Autodesk Inventor part; units mm, degrees
ref_plane "YZ Plane" through (0, 0, 0) normal (1, 0, 0) x (0, 1, 0)
ref_plane "XZ Plane" through (0, 0, 0) normal (0, 1, 0) x (-1, 0, 0)
ref_plane "XY Plane" through (0, 0, 0) normal (0, 0, 1) x (1, 0, 0)
sketch "Sketch1" plane through (0, 0, 0) normal (1, 0, 0) x (0, 1, 0)
  arc A0 (0, -15.5) -> (0, 15.5) centre (0, 0) ccw
  line L0 (0, -15.5) -> (-10, -15.5)
  line L1 (0, -15.5) -> (0, -16.75)
  arc A1 (0, -16.75) -> (0, 16.75) centre (0, 0) ccw
  line L2 (0, -16.75) -> (-10, -16.75)
  line L3 (-10, -15.5) -> (-10, -27.5)
  line L4 (-10, -16.75) -> (-8.75, -16.75)
  line L5 (-8.75, -27.5) -> (-8.75, -28.75)
  line L6 (-15.5, 0) -> (-15.5, -28.75)
  line L7 (-8.75, -27.5) -> (-8.75, -16.75)
  line L8 (0, 0) -> (-6.7436, 0)
  line L9 (0, 15.5) -> (-10, 15.5)
  line L10 (0, 16.75) -> (-8.75, 16.75)
  line L11 (-10, 15.5) -> (-10, 27.5)
  line L12 (-8.75, 27.5) -> (-8.75, 28.75)
  line L13 (-15.5, 0) -> (-15.5, 28.75)
  line L14 (-8.75, 27.5) -> (-8.75, 16.75)
  line L15 (-10, -27.5) -> (-10, -28.5)
  line L16 (-10, -28.5) -> (-15.5, -28.5)
  line L17 (-15.5, -28.5) -> (-15.5, -29.75)
  line L18 (-15.5, -29.75) -> (-8.75, -29.75)
  line L19 (-8.75, -29.75) -> (-8.75, -28.75)
  line L20 (-8.75, 27.5) -> (-8.75, 28.75)
  line L21 (-10, 27.5) -> (-10, 28.5)
  line L22 (-10, 28.5) -> (-15.5, 28.5)
  line L23 (-15.5, 28.5) -> (-15.5, 29.75)
  line L24 (-15.5, 29.75) -> (-8.75, 29.75)
  line L25 (-8.75, 29.75) -> (-8.75, 28.75)
  point P0 (-10, 16.75)
  dimension "d0" = 31
  dimension "d1" = 10
  dimension "d2" = 1.25
  dimension "d3" = 12
  dimension "d4" = 1.25
  dimension "d5" = 1.25
  dimension "d6" = 1
  dimension "d7" = 1.25
extrude "Extrusion1" add sketch "Sketch1" along normal blind 35 contours L1 L2 L3 L0 | A0 L9 L11 L21 L22 L13 L23 L24 L25 L12 L14 L10 A1 L1 | L2 L7 L5 L19 L18 L17 L6 L16 L15 L3
sketch "Sketch2" plane through (35, 0, 0) normal (1, 0, 0) x (0, 0, -1)
  line L0 (29.75, -8.75) -> (16.75, -8.75)
  line L1 (16.75, -8.75) -> (16.75, 0)
  arc A0 (16.75, 0) -> (-16.75, 0) centre (0, 0) ccw
  line L2 (-16.75, 0) -> (-16.75, -8.75)
  line L3 (-16.75, -8.75) -> (-29.75, -8.75)
  line L4 (-29.75, -8.75) -> (-29.75, -15.5)
  line L5 (-29.75, -15.5) -> (-28.5, -15.5)
  line L6 (-28.5, -15.5) -> (-28.5, -10)
  line L7 (-28.5, -10) -> (-15.5, -10)
  line L8 (-15.5, -10) -> (-15.5, 0)
  arc A1 (15.5, 0) -> (-15.5, 0) centre (0, 0) ccw
  line L9 (15.5, 0) -> (15.5, -10)
  line L10 (15.5, -10) -> (28.5, -10)
  line L11 (28.5, -10) -> (28.5, -15.5)
  line L12 (28.5, -15.5) -> (29.75, -15.5)
  line L13 (29.75, -15.5) -> (29.75, -8.75)
  line L14 (-28.5, -15.5) -> (-28.5, -10)
  line L15 (-28.5, -15.5) -> (0, -15.5)
  line L16 (0, -15.5) -> (0, 27.5)
  line L17 (0, 27.5) -> (0, 6)
  line L18 (21.5, 6) -> (21.5, -15.5)
  line L19 (21.5, -15.5) -> (22.75, -15.5)
  line L20 (22.75, -15.5) -> (22.75, 6)
  line L21 (-21.5, 6) -> (-21.5, -15.5)
  line L22 (-21.5, -15.5) -> (-22.75, -15.5)
  line L23 (-22.75, -15.5) -> (-22.75, 6)
  arc A2 (22.75, 6) -> (-22.75, 6) centre (0, 6) ccw
  arc A3 (-17.3205, -8.75) -> (-16.1729, -10) centre (0, 6) ccw
  arc A4 (16.1729, -10) -> (17.3205, -8.75) centre (0, 6) ccw
  arc A5 (-16.75, -7.4792) -> (-15.5, -8.8997) centre (0, 6) ccw
  arc A6 (15.5, -8.8997) -> (16.75, -7.4792) centre (0, 6) ccw
  arc A7 (21.5, 6) -> (-21.5, 6) centre (0, 6) ccw
  dimension "d10" = 43
  dimension "d11" = 21.5
  dimension "d12" = 1.25
extrude "Extrusion2" add sketch "Sketch2" along normal blind 103 contours L18 A7 L21 L3 L23 A2 L20 L0 | L0 L20 L10 L18 | L10 L20 L19 L18 | L3 L21 L7 L23 | L7 L21 L15 L23
sketch "Sketch3" plane through (35, 0, 0) normal (-1, 0, 0) x (0, 0, 1)
  line L0 (-22.75, -8.75) -> (-21.5, -8.75)
  line L1 (-21.5, 6) -> (-21.5, -8.75)
  arc A0 (21.5, 6) -> (-21.5, 6) centre (0, 6) ccw
  line L2 (21.5, -8.75) -> (21.5, 6)
  line L3 (21.5, -8.75) -> (22.75, -8.75)
  line L4 (22.75, 6) -> (22.75, -8.75)
  arc A1 (22.75, 6) -> (-22.75, 6) centre (0, 6) ccw
  line L5 (-22.75, -8.75) -> (-22.75, 6)
  line L6 (-29.75, -8.75) -> (-16.75, -8.75)
  line L7 (-29.75, -15.5) -> (-29.75, -8.75)
  line L8 (-28.5, -15.5) -> (-29.75, -15.5)
  line L9 (-28.5, -10) -> (-28.5, -15.5)
  line L10 (-15.5, -10) -> (-28.5, -10)
  line L11 (-15.5, 0) -> (-15.5, -10)
  arc A2 (15.5, 0) -> (-15.5, 0) centre (0, 0) ccw
  line L12 (15.5, -10) -> (15.5, 0)
  line L13 (28.5, -10) -> (15.5, -10)
  line L14 (28.5, -15.5) -> (28.5, -10)
  line L15 (29.75, -15.5) -> (28.5, -15.5)
  line L16 (29.75, -8.75) -> (29.75, -15.5)
  line L17 (16.75, -8.75) -> (29.75, -8.75)
  line L18 (16.75, 0) -> (16.75, -8.75)
  arc A3 (16.75, 0) -> (-16.75, 0) centre (0, 0) ccw
  line L19 (-16.75, -8.75) -> (-16.75, 0)
extrude "Extrusion3" add sketch "Sketch3" along normal blind 1.25 contours L5 A1 L4 L3 L2 A0 L1 L0 | L1 A0 L2 L17 L18 A3 L19 L6
sketch "Sketch4" plane through (0, -8.75, 29.75) normal (0, 1, 0) x (1, 0, 0)
  line L0 (33.75, 7) -> (33.75, 13)
  line L1 (0, 13) -> (33.75, 13)
  line L2 (0, 13) -> (0, 0)
  line L3 (0, 0) -> (35, 0)
  line L4 (35, 7) -> (35, 0)
  line L5 (35, 7) -> (33.75, 7)
  line L6 (33.75, 46.5) -> (33.75, 52.5)
  line L7 (33.75, 52.5) -> (35, 52.5)
  line L8 (35, 59.5) -> (35, 52.5)
  line L9 (0, 59.5) -> (35, 59.5)
  line L10 (0, 59.5) -> (0, 46.5)
  line L11 (0, 46.5) -> (33.75, 46.5)
  line L12 (33.75, 7) -> (33.75, 0)
  line L13 (0, 0) -> (35, 0)
  line L14 (33.75, 52.5) -> (33.75, 59.5)
  line L15 (0, 59.5) -> (35, 59.5)
  point P0 (0, 29.75)
extrude "Extrusion4" cut sketch "Sketch4" against normal through all contours L5 L4 L3 L12 | L14 L9 L8 L7
sketch "Sketch5" plane through (35, 0, 0) normal (-1, 0, 0) x (0, 0, 1)
  line L0 (-21.5, -10) -> (-22.75, -10)
  line L1 (-22.75, -15.5) -> (-22.75, -10)
  line L2 (-21.5, -15.5) -> (-22.75, -15.5)
  line L3 (-21.5, -10) -> (-21.5, -15.5)
  line L4 (22.75, -10) -> (21.5, -10)
  line L5 (21.5, -15.5) -> (21.5, -10)
  line L6 (22.75, -15.5) -> (21.5, -15.5)
  line L7 (22.75, -10) -> (22.75, -15.5)
  point P0 (0, 0)
extrude "Extrusion5" add sketch "Sketch5" along normal blind 2.5
sketch "Sketch6" plane through (138, -15.5, 22.75) normal (0, 0, 1) x (1, 0, 0)
  line L0 (-104.25, 0) -> (-104.25, 6.75)
  line L1 (-138, 6.75) -> (-104.25, 6.75)
  line L2 (-138, 6.75) -> (-138, 0)
  line L3 (-138, 0) -> (-104.25, 0)
  line L4 (-105.5, 0) -> (-105.5, 5.5)
  line L5 (-105.5, 5.5) -> (-104.25, 5.5)
  point P0 (-138, 15.5)
extrude "Extrusion6" add sketch "Sketch6" along normal blind 7 contours L3 L4 L5 L0
sketch "Sketch7" plane through (138, -15.5, -22.75) normal (0, 0, -1) x (-1, 0, 0)
  line L0 (104.25, 6.75) -> (104.25, 0)
  line L1 (105.5, 5.5) -> (105.5, 0)
  line L2 (103, 5.5) -> (105.5, 5.5)
  line L3 (105.5, 0) -> (0, 0)
  point P0 (138, 15.5)
  point P1 (104.25, 5.5)
extrude "Extrusion7" add sketch "Sketch7" along normal blind 7
sketch "Sketch8" plane through (138, 0, 0) normal (1, 0, 0) x (0, 0, -1)
  line L0 (-22.75, 6) -> (-22.75, -15.5)
  line L1 (-22.75, -15.5) -> (-21.5, -15.5)
  line L2 (-21.5, -15.5) -> (-21.5, 6)
  arc A0 (21.5, 6) -> (-21.5, 6) centre (0, 6) ccw
  line L3 (21.5, 6) -> (21.5, -15.5)
  line L4 (21.5, -15.5) -> (22.75, -15.5)
  line L5 (22.75, -15.5) -> (22.75, 6)
  arc A1 (22.75, 6) -> (-22.75, 6) centre (0, 6) ccw
  line L6 (-22.75, -15.5) -> (22.75, -15.5)
  line L7 (-21.5, -15.5) -> (-28.5, -15.5)
  point P0 (0, 0)
extrude "Extrusion8" add sketch "Sketch8" along normal blind 1.25
sketch "Sketch9" plane through (33.75, -8.75, 22.75) normal (0, 0, 1) x (1, 0, 0)
  line L0 (0, 0) -> (0, -6.75)
  line L1 (0, -6.75) -> (105.5, -6.75)
  line L2 (105.5, 14.75) -> (105.5, -6.75)
  line L3 (105.5, 14.75) -> (0, 14.75)
  line L4 (0, 0) -> (0, 14.75)
  line L5 (105.5, -6.75) -> (96.5, -6.75)
  line L6 (-1.25, -6.75) -> (104.25, -6.75)
  line L7 (96.5, -6.75) -> (96.5, -5.5)
  line L8 (96.5, -5.5) -> (88.5, -5.5)
  line L9 (88.5, -5.5) -> (88.5, -6.75)
  point P0 (-33.75, 8.75)
  dimension "d27" = 9
  dimension "d28" = 1.25
  dimension "d29" = 8
extrude "Extrusion9" add sketch "Sketch9" along normal blind 8 contours L9 L8 L7 L1
sketch "Sketch10" plane through (33.75, -8.75, -22.75) normal (0, 0, -1) x (-1, 0, 0)
  line L0 (-88.5, -6.75) -> (-96.5, -6.75)
  line L1 (-88.5, -5.5) -> (-88.5, -6.75)
  line L2 (-88.5, -6.75) -> (-96.5, -6.75)
  line L3 (-96.5, -6.75) -> (-96.5, -5.5)
  line L4 (-96.5, -5.5) -> (-88.5, -5.5)
  point P0 (33.75, 8.75)
extrude "Extrusion10" add sketch "Sketch10" along normal blind 8
sketch "Sketch11" plane through (122.25, -14.25, -22.75) normal (0, 1, 0) x (1, 0, 0)
  line L0 (8, 0) -> (0, 0)
  line L1 (8, 0) -> (8, 8)
  line L2 (0, 8) -> (8, 8)
  line L3 (0, 0) -> (0, 8)
  line L4 (0, -45.5) -> (8, -45.5)
  line L5 (0, -45.5) -> (0, -53.5)
  line L6 (8, -53.5) -> (0, -53.5)
  line L7 (8, -45.5) -> (8, -53.5)
  line L8 (0, -45.5) -> (0, -53.5)
  line L9 (0, -53.5) -> (4, -53.5)
  line L10 (0, -53.5) -> (8, -53.5)
  line L11 (4, -53.5) -> (4, -49.5)
  circle A0 centre (4, -49.5) radius 1.8
  line L12 (0, 8) -> (8, 8)
  line L13 (8, 8) -> (4, 8)
  line L14 (8, 8) -> (12, 8) construction
  line L15 (4, 8) -> (4, 4)
  line L16 (0, 0) -> (0, 8)
  circle A1 centre (4, 4) radius 1.8
  point P0 (-122.25, -22.75)
  dimension "d34" = 4
  dimension "d35" = 3.6
  dimension "d36" = 4
  dimension "d37" = 180
  dimension "d38" = 3.6
extrude "Extrusion11" cut sketch "Sketch11" against normal blind 8 contours A1 | A0
fillet "Fillet1" radius 1 6 edges at (130.25, -14.875, 22.75) (126.25, -14.25, 22.75) (122.25, -14.875, 22.75) (130.25, -14.875, -22.75) (126.25, -14.25, -22.75) (122.25, -14.875, -22.75)
fillet "Fillet2" radius 2 3 edges at (33.75, -4.375, -16.75) (33.75, -4.375, 16.75) (33.75, 16.75, 0)
sketch "Sketch12" plane through (0, -8.75, -16.75) normal (0, 1, 0) x (1, 0, 0)
  arc A0 (31.75, 0) -> (33.75, 2) centre (31.75, 2) ccw
  line L0 (33.75, 2) -> (33.75, 6)
  line L1 (33.75, 6) -> (33.75, 13)
  line L2 (0, 13) -> (33.75, 13)
  line L3 (0, 13) -> (0, 0)
  line L4 (0, 0) -> (31.75, 0)
  arc A1 (33.75, -35.5) -> (31.75, -33.5) centre (31.75, -35.5) ccw
  line L5 (0, -33.5) -> (31.75, -33.5)
  line L6 (0, -33.5) -> (0, -46.5)
  line L7 (0, -46.5) -> (33.75, -46.5)
  line L8 (33.75, -46.5) -> (33.75, -39.5)
  line L9 (33.75, -39.5) -> (33.75, -35.5)
  line L10 (0, 13) -> (-2.5, 13)
  line L11 (-2.5, 13) -> (4, 13)
  line L12 (0, 13) -> (33.75, 13)
  line L13 (4, 13) -> (4, 8.75)
  line L14 (4, 8.75) -> (4, 4.4)
  circle A2 centre (4, 4.4) radius 2.55
  line L15 (0, 0) -> (0, -16.75)
  line L16 (0, -16.75) -> (16.875, -16.75)
  circle A3 centre (4, -37.9) radius 2.55
  dimension "d43" = 2.5
  dimension "d44" = 6.5
  dimension "d45" = 4.25
  dimension "d46" = 4.35
  dimension "d47" = 5.1
extrude "Extrusion12" cut sketch "Sketch12" against normal blind 8 contours A2 | A3
properties part number "carcasa_motores"
Verification items for the finished model (mm, model axes). A direction names the side the tool comes from. Coordinates: 2 decimals unless noted, no trailing zeros. Loops run counter-clockwise (first coordinate to the right, second up) from the corner with the lowest first, then second, coordinate; pieces in that order, holes last. Notation, with made-up numbers: (34, -5.75) -> (72, -5.75) arc R19 ccw to (72, 4.25) -> close; hole circle Ø7 at (64, 45). An arc over 180 degrees is marked (long way). Answer as a JSON object with one key per item and string values. Group by question number.
Item 1: Sectioned sample at B-B on x = 4. Record the boundary of the cut face in (y, z), plus the area to 3 significant figures.
Item 2: Sectioned sample at A-A on z = -26.75. Record the boundary of the cut face in (x, y), plus the area to 3 significant figures.
Item 3: Sectioned sample at C-C on y = -3. Record the boundary of the cut face in (x, z), plus the area to 3 significant figures.
Item 4: Scan lines: probe 1 along X at (y, z) = (-9.15, -21.15); probe 2 along Z at (x, y) = (4, -9.7); probe 3 along Z at (x, y) = (126, -15). Record each from-to range of solid material in increasing order.
Item 5: Sectioned sample at D-D on z = 0. Record the boundary of the cut face in (x, y), plus the area to 3 significant figures.
Item 6: Mould release check, pull along X, two halves, no side actions. Record for faces 4 (the flat face through (33.75, -12, -26)), 5 (the cylindrical face through (87.238, 28.744, -0.5)), 6 (the flat face through (139.25, 7, 0)): +X half, -X half, draft (parallel to the pull), parting line (faces both ways), or undercut.
Item 7: Tool access check on faces 1 (the flat face through (17, -12, 29.75)), 2 (the flat face through (17, -5, 15.5)), 3 (the flat face through (16, -4, 16.75)). Record the directions out of +Z, -Z, +X, -X, +Y, -Y that give a thin tool (end or side, any length) a straight path to the whole face; none if there is none.
Item 8: Depth check by flat-ended pin: pin 1 (1 mm diameter, centred on y = 18, z = -9, fed in from -X); pin 2 (1.4 mm diameter, centred on y = -15, z = 28, fed in from +X); pin 3 (4 mm diameter, centred on x = 124, z = 11, fed in from +Y). Enter the tip coordinate at first touch or a pass-through.
Evaluation:
{
 "1": {"outline": "(-15.5, -29.75) -> (-8.75, -29.75) -> (-8.75, -23.7) -> (-10, -23.7) -> (-10, -28.5) -> (-15.5, -28.5) -> close; (-15.5, 28.5) -> (-10, 28.5) -> (-10, 23.7) -> (-8.75, 23.7) -> (-8.75, 29.75) -> (-15.5, 29.75) -> close; (-10, -18.6) -> (-8.75, -18.6) -> (-8.75, -16.75) -> (0, -16.75) arc R16.75 ccw to (0, 16.75) -> (-8.75, 16.75) -> (-8.75, 18.6) -> (-10, 18.6) -> (-10, 15.5) -> (0, 15.5) arc R15.5 cw to (0, -15.5) -> (-10, -15.5) -> close", "area": "122 mm²"},
 "2": {"outline": "(0, -10) -> (32.5, -10) -> (32.5, -15.5) -> (33.75, -15.5) -> (33.75, -8.75) -> (0, -8.75) -> close; (122.25, -15.5) -> (124.45, -15.5) -> (124.45, -14.25) -> (122.25, -14.25) -> close; (128.05, -15.5) -> (130.25, -15.5) -> (130.25, -14.25) -> (128.05, -14.25) -> close", "area": "54.6 mm²"},
 "3": {"outline": "(0, -16.75) -> (31.75, -16.75) arc R2 cw to (33.75, -18.75) -> (33.75, -22.75) -> (139.25, -22.75) -> (139.25, 22.75) -> (33.75, 22.75) -> (33.75, 18.75) arc R2 cw to (31.75, 16.75) -> (0, 16.75) -> (0, 15.5) -> (35, 15.5) -> (35, 21.5) -> (138, 21.5) -> (138, -21.5) -> (35, -21.5) -> (35, -15.5) -> (0, -15.5) -> close", "area": "419 mm²"},
 "4": {"probe 1": "x = 0 to 1.45, 6.55 to 35, 138 to 139.25", "probe 2": "z = -29.75 to -23.7, -18.6 to -15.5, 15.5 to 18.6, 23.7 to 29.75", "probe 3": "z = -30.75 to -28.53, -24.97 to -21.5, 21.5 to 24.97, 28.53 to 30.75"},
 "5": {"outline": "(0, 15.5) -> (35, 15.5) -> (35, 27.5) -> (138, 27.5) -> (138, -15.5) -> (139.25, -15.5) -> (139.25, 28.75) -> (33.75, 28.75) -> (33.75, 18.75) arc R2 cw to (31.75, 16.75) -> (0, 16.75) -> close", "area": "244 mm²"},
 "6": {"face 4": "undercut", "face 5": "draft", "face 6": "+X half"},
 "7": {"face 1": "+Z, -X, +Y, -Y", "face 2": "-X, -Y", "face 3": "+Z, -X, +Y"},
 "8": {"pin 1": "stops at x = 33.75", "pin 2": "stops at x = 130.25", "pin 3": "stops at y = 26.89"}
}
